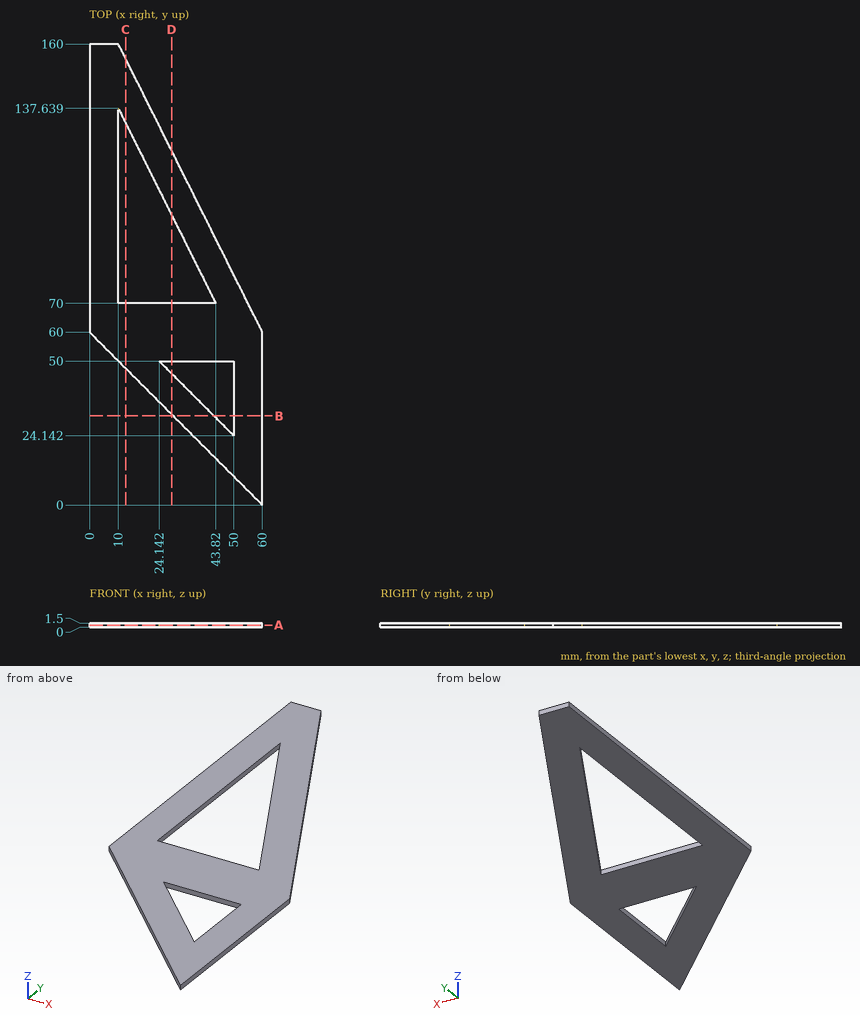
Can you work these out from the drawing? Everything is in mm from the part's minimum corner. Coordinates: 2 decimals unless noted, no trailing zeros. Loops run counter-clockwise (first coordinate to the right, second up) from the corner with the lowest first, then second, coordinate; pieces in that order, holes last.
1) For pin 1 (0.8 mm diameter, centred on x = 29.5, z = 1, fed in from +Y); pin 2 (0.8 mm diameter, centred on x = 33.5, z = 0.5, fed in from -Y), each with a flat end and sliding along its axis, tell me the tip position at first contact or that it passes through.
2) Imagine slicing it at B-B on y = 31. List the corners of the cut face in (x, z) for me.
3) I need wall thicknesses on probe 1 along Y at (x, z) = (36, 1.2) (1 decimal); probe 2 along Y at (x, z) = (34, 0.55) (1 decimal); probe 3 along X at (y, z) = (105, 0.15). Which ranges of each line are inside material? Lowest first, please.
4) Imagine slicing it at D-D on x = 28.5. List the corners of the cut face in (y, z) for me.
5) Imagine slicing it at A-A on z = 0.8. List the corners of the cut face in (x, y) for me.
6) Imagine slicing it at C-C on x = 12.5. List the corners of the cut face in (y, z) for me.
Completed:
1. pin 1: stops at y = 121.8
1. pin 2: stops at y = 26.1
2. outline: (29, 0) - (43.14, 0) - (43.14, 1.5) - (29, 1.5) - close; (50, 0) - (60, 0) - (60, 1.5) - (50, 1.5) - close
3. probe 1: y = 24 to 38.1, 50 to 70, 85.6 to 108
3. probe 2: y = 26 to 40.1, 50 to 70, 89.6 to 112
3. probe 3: x = 0 to 10, 26.32 to 37.5
4. outline: (31.5, 0) - (45.64, 0) - (45.64, 1.5) - (31.5, 1.5) - close; (50, 0) - (70, 0) - (70, 1.5) - (50, 1.5) - close; (100.64, 0) - (123, 0) - (123, 1.5) - (100.64, 1.5) - close
5. outline: (0, 60) - (60, 0) - (60, 60) - (10, 160) - (0, 160) - close; hole (10, 70) - (43.82, 70) - (10, 137.64) - close; hole (24.14, 50) - (50, 24.14) - (50, 50) - close
6. outline: (47.5, 0) - (70, 0) - (70, 1.5) - (47.5, 1.5) - close; (132.64, 0) - (155, 0) - (155, 1.5) - (132.64, 1.5) - close
